The listing builds one solid part. Answer for the finished solid, in the listing's coordinates (mm). Round coordinates to 2 decimals unless told otherwise and drop trailing zeros. Write each loop counter-clockwise with the first axis right and the second up, starting at its lowest first coordinate (ties: lowest second). Pieces come first, ordered by that corner, then holes.
(1) Find the intervals of material crossed by probe 1 along Y at (x, z) = (0, 8.25); probe 2 along X at (y, z) = (-6, 14); probe 3 along X at (y, z) = (86, 12), in increasing order.
(2) A cutting plane is placed at A-A, the plane y = 0. Give the vertices of the cut face in (x, z), and give its area (3 significant figures).
(3) A cutting plane is placed at C-C, the plane z = 9.25. Give the vertices of the cut face in (x, y).
(4) Each of these flat-tipped pins is pushed along its axis until it touches: pin 1 Ø10 at (y, z) = (55.5, 12.5) entering from -X; pin 2 Ø5 at (x, y) = (85.5, 23.5) entering from +Z; pin 3 Ø6 at (x, z) = (61.5, 7) entering from +Y; pin 4 Ø10 at (x, z) = (28.5, 16) entering from -Y. Where does it stop, or does it pass through?
(5) A cutting plane is placed at B-B, the plane x = 0. Give the vertices of the cut face in (y, z), and give its area (3 significant figures).
from build123d import *

# Parameters (mm, degrees)
F0_W     = 177.8
F0_H     = 228.6
F1_DEPTH = 19.05
F2_W     = 6.35
F2_H     = 12.7
F3_DEPTH = 254
F4_R     = 63.5
F4_R_2   = 31.75
F5_DEPTH = 25.4
F6_R     = 6.35


with BuildPart() as f1:
    # F0 (on Top) → F1 (new body)
    with BuildSketch(Plane.XY):
        Rectangle(F0_W, F0_H)
    extrude(amount=F1_DEPTH)

    # F2 (on face) → F3 (cut)
    with BuildSketch(Plane.XZ.offset(114.3)):
        with Locations((85.725, 12.7)):
            Rectangle(F2_W, F2_H)
        with Locations((-85.725, 12.7)):
            Rectangle(F2_W, F2_H)
    extrude(amount=-F3_DEPTH, mode=Mode.SUBTRACT)

    # F4 (on face) → F5 (cut)
    with BuildSketch(Plane.XY.offset(19.05)):
        with Locations((0, -114.3)):
            Circle(F4_R)
        with Locations((0, 114.3)):
            Circle(F4_R)
        Circle(F4_R_2)
    extrude(amount=-F5_DEPTH, mode=Mode.SUBTRACT)

    # F6
    f6_edges = [f1.edges().sort_by_distance(p)[0] for p in [
        (0, 50.8, 0),
        (-31.75, 0, 0),
        (0, -50.8, 0),
        (0, 50.8, 19.05),
        (-31.75, 0, 19.05),
        (0, -50.8, 19.05),
    ]]
    fillet(f6_edges, radius=F6_R)


solid = f1.part
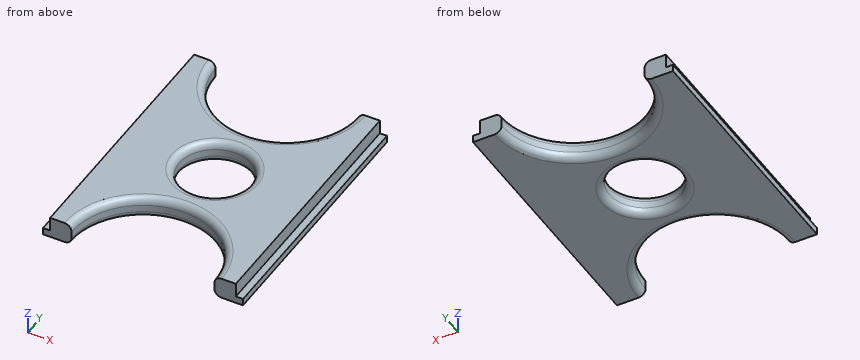
Solutions:
1. probe 1: y = -50.8 to -31.75, 31.75 to 50.8
1. probe 2: x = -82.55 to -31.31, 31.31 to 82.55
1. probe 3: x = -82.55 to -56.85, 56.85 to 82.55
2. outline: (-88.9, 0) - (-38.1, 0) arc R6.35 ccw to (-31.75, 6.35) - (-31.75, 12.7) arc R6.35 ccw to (-38.1, 19.05) - (-82.55, 19.05) - (-82.55, 6.35) - (-88.9, 6.35) - close; (31.75, 6.35) arc R6.35 ccw to (38.1, 0) - (88.9, 0) - (88.9, 6.35) - (82.55, 6.35) - (82.55, 19.05) - (38.1, 19.05) arc R6.35 ccw to (31.75, 12.7) - close
2. area: 1,980 mm2
3. outline: (-82.55, -114.3) - (-63.5, -114.3) arc R63.5 cw to (63.5, -114.3) - (82.55, -114.3) - (82.55, 114.3) - (63.5, 114.3) arc R63.5 cw to (-63.5, 114.3) - (-82.55, 114.3) - close; hole circle Ø63.5 at (0, 0)
4. pin 1: stops at x = -82.55
4. pin 2: stops at z = 6.35
4. pin 3: stops at y = 114.3
4. pin 4: stops at y = -59.94
5. outline: (-50.8, 6.35) arc R6.35 ccw to (-44.45, 0) - (-38.1, 0) arc R6.35 ccw to (-31.75, 6.35) - (-31.75, 12.7) arc R6.35 ccw to (-38.1, 19.05) - (-44.45, 19.05) arc R6.35 ccw to (-50.8, 12.7) - close; (31.75, 6.35) arc R6.35 ccw to (38.1, 0) - (44.45, 0) arc R6.35 ccw to (50.8, 6.35) - (50.8, 12.7) arc R6.35 ccw to (44.45, 19.05) - (38.1, 19.05) arc R6.35 ccw to (31.75, 12.7) - close
5. area: 657 mm2
